from build123d import *

# Parameters (mm, degrees)
BOSS_EXTRUDE1_DEPTH = 20
CUT_EXTRUDE1_DEPTH  = 15
BOSS_EXTRUDE2_DEPTH = 5
CUT_EXTRUDE2_REACH  = 90.178
SKETCH2_R           = 2.1
CUT_EXTRUDE3_REACH  = 90.178
SKETCH3_R           = 2.1
FILLET2_R           = 84
FILLET3_R           = 3.5
FILLET4_R           = 1


with BuildPart() as part:
    # Sketch1 → Boss-Extrude1 (new body)
    with BuildSketch(Plane.XY):
        Polygon((41.8365, 5), (5, 5), (5, 75), (0, 75), (0, 0), (41.8365, 0), align=None)
    extrude(amount=BOSS_EXTRUDE1_DEPTH)

    # Sketch1<3> → Cut-Extrude1 (cut)
    with BuildSketch(Plane.XY):
        Polygon((41.8365, 5), (5, 5), (5, 75), (3, 75), (3, 3), (41.8365, 3), align=None)
    extrude(amount=CUT_EXTRUDE1_DEPTH, mode=Mode.SUBTRACT)

    # Sketch1<4> → Boss-Extrude2 (add)
    with BuildSketch(Plane.XY):
        Polygon((41.8365, 5), (5, 5), (5, 75), (3, 75), (3, 3), (41.8365, 3), align=None)
    extrude(amount=BOSS_EXTRUDE2_DEPTH)

    # Sketch2 → Cut-Extrude2 (cut, up to next)
    with BuildSketch(Plane.XZ, mode=Mode.PRIVATE) as cut_extrude2_sk1:
        with Locations(Location((11.8365, 10, 0), (0, 0, 270))):
            Circle(SKETCH2_R)
    cut_extrude2_tool1 = extrude(cut_extrude2_sk1.sketch, amount=-CUT_EXTRUDE2_REACH, mode=Mode.PRIVATE) & part.part
    add(cut_extrude2_tool1.solids().sort_by_distance((11.8365, 0, 10))[0], mode=Mode.SUBTRACT)

    # Sketch3 → Cut-Extrude3 (cut, up to next)
    with BuildSketch(Plane.ZY, mode=Mode.PRIVATE) as cut_extrude3_sk1:
        with Locations((10, 25)):
            Circle(SKETCH3_R)
    cut_extrude3_tool1 = extrude(cut_extrude3_sk1.sketch, amount=-CUT_EXTRUDE3_REACH, mode=Mode.PRIVATE) & part.part
    # Sketch3 → Cut-Extrude3 (cut, up to next)
    with BuildSketch(Plane.ZY, mode=Mode.PRIVATE) as cut_extrude3_sk2:
        with Locations((10, 50)):
            Circle(SKETCH3_R)
    cut_extrude3_tool2 = extrude(cut_extrude3_sk2.sketch, amount=-CUT_EXTRUDE3_REACH, mode=Mode.PRIVATE) & part.part
    add(cut_extrude3_tool1.solids().sort_by_distance((0, 25, 10))[0], mode=Mode.SUBTRACT)
    add(cut_extrude3_tool2.solids().sort_by_distance((0, 50, 10))[0], mode=Mode.SUBTRACT)

    # Fillet2
    # the kernel refuses this fillet: 84 mm, written as the material it adds along each edge
    with BuildSketch(Plane(origin=(5, 5, -158.774355627), x_dir=(1, 0, 0), z_dir=(0, 0, 1))) as fillet2_piece_1_section:
        with BuildLine():
            CenterArc((84, 69.509742251), FILLET2_R, 180, 55.842464398)
            Line((0, 69.509742251), (-1.68, 69.509742251))
            Line((-1.68, 69.509742251), (-1.68, 0))
            Line((-1.68, 0), (0, -1.68))
            ThreePointArc((0, -1.68), (18.41825, -1.68), (35.89323, -1.390194845))
            Line((35.89323, -1.390194845), (36.8365, 0))
        make_face()
    fillet2_piece_1 = extrude(amount=178.774355627, mode=Mode.PRIVATE)
    fillet2_piece_1 = split(fillet2_piece_1, bisect_by=Plane(origin=(14.491057498, 22.671022952, 0), z_dir=(0, 0, 1)), keep=Keep.TOP, mode=Mode.PRIVATE)
    fillet2_piece_1 = split(fillet2_piece_1, bisect_by=Plane(origin=(14.491057498, 22.671022952, 5), z_dir=(0, 0, -1)), keep=Keep.TOP, mode=Mode.PRIVATE)
    add(fillet2_piece_1)
    with BuildSketch(Plane(origin=(5, 5, 15), x_dir=(1, 0, 0), z_dir=(0, 0, 1)), Plane(origin=(5, 5, 0), x_dir=(1, 0, 0), z_dir=(0, 0, 1))) as fillet2_piece_2:
        with BuildLine():
            CenterArc((84, 69.509742251), FILLET2_R, 180, 55.842464398)
            Line((0, 69.509742251), (-1.68, 69.509742251))
            Line((-1.68, 69.509742251), (-1.68, 0))
            Line((-1.68, 0), (0, -1.68))
            ThreePointArc((0, -1.68), (18.41825, -1.68), (35.89323, -1.390194845))
            Line((35.89323, -1.390194845), (36.8365, 0))
        make_face()
    extrude(amount=5)
    with BuildSketch(Plane(origin=(5, 5, 0), x_dir=(1, 0, 0), z_dir=(0, 0, 1))) as fillet2_piece_3_section:
        with BuildLine():
            CenterArc((84, 69.509742251), FILLET2_R, 180, 55.842464398)
            Line((0, 69.509742251), (-1.68, 69.509742251))
            Line((-1.68, 69.509742251), (-1.68, 0))
            Line((-1.68, 0), (0, -1.68))
            ThreePointArc((0, -1.68), (18.41825, -1.68), (35.89323, -1.390194845))
            Line((35.89323, -1.390194845), (36.8365, 0))
        make_face()
    fillet2_piece_3 = extrude(amount=178.774355627, mode=Mode.PRIVATE)
    fillet2_piece_3 = split(fillet2_piece_3, bisect_by=Plane(origin=(14.491057498, 22.671022952, 15), z_dir=(0, 0, 1)), keep=Keep.TOP, mode=Mode.PRIVATE)
    fillet2_piece_3 = split(fillet2_piece_3, bisect_by=Plane(origin=(14.491057498, 22.671022952, 20), z_dir=(0, 0, -1)), keep=Keep.TOP, mode=Mode.PRIVATE)
    add(fillet2_piece_3)

    # Fillet3
    # the kernel refuses this fillet: 3.5 mm, written as the material it adds along each edge
    with BuildSketch(Plane(origin=(3, 3, 5), x_dir=(1, 0, 0), z_dir=(0, 0, 1))) as fillet3_piece_1:
        with BuildLine():
            CenterArc((FILLET3_R, FILLET3_R), FILLET3_R, 180, 90)
            Line((0, FILLET3_R), (-FILLET3_R * 0.02, FILLET3_R))
            Line((-FILLET3_R * 0.02, FILLET3_R), (-FILLET3_R * 0.02, -FILLET3_R * 0.02))
            Line((-FILLET3_R * 0.02, -FILLET3_R * 0.02), (FILLET3_R, -FILLET3_R * 0.02))
            Line((FILLET3_R, -FILLET3_R * 0.02), (FILLET3_R, 0))
        make_face()
    extrude(amount=10)
    # the kernel refuses this fillet: 3.5 mm, written as the material it takes off along each edge
    with BuildSketch(Plane(origin=(5, 75, -20.689329277), x_dir=(-1, 0, 0), z_dir=(0, 0, 1))) as fillet3_2_piece_1:
        with BuildLine():
            CenterArc((3.448221546, 3.5), FILLET3_R, 181.971194875, 88.028805125)
            Line((-0.049707316, 3.37961031), (-0.399500202, 3.367571341))
            ThreePointArc((-0.399500202, 3.367571341), (-0.35, 0.490257749), (-0.35, 0))
            Line((-0.35, 0), (0, -0.35))
            Line((0, -0.35), (3.448221546, -0.35))
            Line((3.448221546, -0.35), (3.448221546, 0))
        make_face()
    extrude(amount=46.378658554, mode=Mode.SUBTRACT)
    with BuildSketch(Plane(origin=(41.8365, 5, -10.984244879), x_dir=(0, -1, 0), z_dir=(0, 0, 1))) as fillet3_2_piece_2:
        with BuildLine():
            CenterArc((1.83070748, -3.5), FILLET3_R, 90, 54.618958209)
            Line((-1.022910509, -1.47346), (-1.079982869, -1.4329292))
            ThreePointArc((-1.079982869, -1.4329292), (-0.565023995, -0.699541323), (-0.057924785, 0.039302917))
            Line((-0.057924785, 0.039302917), (0, 0.07))
            Line((0, 0.07), (1.83070748, 0.07))
            Line((1.83070748, 0.07), (1.83070748, 0))
        make_face()
    extrude(amount=26.968489758, mode=Mode.SUBTRACT)
    with BuildSketch(Plane(origin=(41.8365, 5, 4.015755121), x_dir=(-0.8214550012543749, 0.5702733387720094, 0), z_dir=(0, 0, 1))) as fillet3_2_piece_3:
        with BuildLine():
            CenterArc((1.831088838, 3.499800501), FILLET3_R, 214.769288697, 54.618958209)
            Line((-1.044003667, 1.503843815), (-1.101505517, 1.463924681))
            Line((-1.101505517, 1.463924681), (-0.05750185, -0.039919134))
            Line((-0.05750185, -0.039919134), (0.000747383, -0.06999601))
            ThreePointArc((0.000747383, -0.06999601), (0.896859839, -0.065212021), (1.792972294, -0.06999601))
            Line((1.792972294, -0.06999601), (1.793719678, 0))
        make_face()
    extrude(amount=26.968489758, mode=Mode.SUBTRACT)

    # Fillet4
    fillet4_edges = [part.edges().sort_by_distance(p)[0] for p in [
        (0.775889227, 75, 20),
        (41.446394693, 4.775080489, 15),
        (4.461432686, 73.445228071, 15),
        (15.036480531, 34.69268827, 20),
        (41.446394693, 4.775080489, 20),
        (3.983715551, 74.017078059, 20),
        (0.775889227, 75, 0),
        (41.8365, 1.58464626, 20),
        (41.8365, 3.08464626, 15),
        (41.8365, 3, 10),
        (41.8365, 3.08464626, 5),
        (41.8365, 1.58464626, 0),
        (15.036480531, 34.69268827, 0),
        (41.446394693, 4.775080489, 0),
        (3.983715551, 74.017078059, 0),
        (15.036480531, 34.69268827, 5),
        (41.446394693, 4.775080489, 5),
        (4.461432686, 73.445228071, 5),
        (15.036480531, 34.69268827, 15),
    ]]
    fillet(fillet4_edges, radius=FILLET4_R)


solid = part.part
Check sheet for the modelled part. Datum: model origin and axes. Units: mm. A direction names the side the tool comes from. Round coordinates to 2 decimals unless told otherwise and drop trailing zeros. Loops run counter-clockwise (first coordinate to the right, second up) from the corner with the lowest first, then second, coordinate; pieces in that order, holes last.
1. Set-up check for faces 5 (the flat face through (12, 23, 5)), 6 (the flat face through (0, 38, 10)): record each of +Z, -Z, +X, -X, +Y, -Y from which the full face is reachable in a straight line by a thin tool's end or side.
2. Mould release check, pull along Z, two halves, no side actions. Record for faces 1 (the flat face through (11, 21, 0)), 2 (the flat face through (12, 21, 20)), 3 (the cylindrical face through (11.9, 1.5, 12.1)), 4 (the flat face through (21, 0, 10)): released by +Z, released by -Z, zero draft, split by the parting line, or undercut.
3. Scan lines: probe 1 along Y at (x, z) = (1.8, 10); probe 2 along Z at (x, y) = (13.5, 8.5); probe 3 along X at (y, z) = (1.1, 10). Record each from-to range of solid material in increasing order.
4. Sectioned sample at A-A on z = 10. Record the boundary of the cut face in (x, y).
5. Gauge pin test, flat ends, axial feed: pin 1 Ø3.5 at (y, z) = (25, 10) entering from -X; pin 2 Ø5 at (x, z) = (24, 9.5) entering from +Y; pin 3 Ø10 at (x, z) = (31.5, 14) entering from +Y; pin 4 Ø6 at (y, z) = (30.5, 9.5) entering from +X. Record the tip position at first contact, or that the pin passes through.
Recorded:
1. face 5: +X, +Y
1. face 6: +Z, -Z, -X, +Y, -Y
2. face 1: released by -Z
2. face 2: released by +Z
2. face 3: undercut
2. face 4: zero draft
3. probe 1: y = 0 to 22.9, 27.1 to 47.9, 52.1 to 74.99
3. probe 2: z = 0 to 5, 15 to 20
3. probe 3: x = 0 to 9.74, 13.94 to 41.84
4. outline: (0, 0) - (9.74, 0) - (9.74, 3) - (6.5, 3) arc R3.5 cw to (3, 6.5) - (3, 22.9) - (0, 22.9) - close; (0, 27.1) - (3, 27.1) - (3, 47.9) - (0, 47.9) - close; (0, 52.1) - (3, 52.1) - (3, 74.69) arc R3.5 ccw to (1.55, 75) - (0, 75) - close; (13.94, 0) - (41.84, 0) - (41.84, 2) arc R1 ccw to (40.84, 3) - (13.94, 3) - close
5. pin 1: passes through
5. pin 2: stops at y = 3
5. pin 3: stops at y = 17.99
5. pin 4: stops at x = 3
